Source: CAD feature listing. Evaluate the final solid. Frame: model axes, mm. A direction names the side the tool comes from. Give positions to 0.01 mm unless a question says otherwise; leave off trailing zeros. Order: outer loops, then holes, each group sorted by start corner. A loop starts at its lowest first (then second) coordinate and runs counter-clockwise, first axis right, second up. Notation, with made-up numbers: M 29.25,55 L 55.25,55 A22 ccw 55.25,93 Z; hole C 6,29.5 d10. An arc over 180 degrees is marked long. Use CSV: the item, a comma, the result in double quotes. Start each with the question number.
Item 1: Ray query, probe 1 along Y at (x, z) = (-76.2, 1.35) (3 decimals); probe 2 along Y at (x, z) = (-78, 2); probe 3 along Y at (x, z) = (-68, 1.45). Return the intervals inside material, ascending. Write a range as from..to.
Item 2: Section query C-C on y = 0. Return loops of the section in (x, z) (3 decimals), and give its area (3 significant figures).
Item 3: Access query for faces 1 (the face through (-7.651, 101.036, 1.252)), 2 (the face through (0.88, 71.75, 1.25)). Directions: +Z, -Z, +X, -X, +Y, -Y. A direction counts if a zero-diameter tool reaches every point of the face in a straight line with its end or side. Return the directions, or none.
Item 4: Section query B-B on x = -76.2. Return loops of the section in (y, z) (3 decimals).
Item 5: Section query A-A on z = 1.15. Return loops of the section in (x, y) (3 decimals), and give its area (3 significant figures).
Item 6: Pull-direction query (X, two-part tool) for faces 3 (the face through (-28, 42, 0)), 4 (the face through (-73.17, 0.95, 1.25)), 5 (the face through (0.304, 44.568, 1.252)); classes: +X half, -X half, draft (parallel to the pull), parting line (faces both ways), or undercut.
Item 7: First-contact query: pin 1 (1 mm diameter, centred on x = -26.5, z = 0.5, fed in from -Y); pin 2 (4 mm diameter, centred on x = -25.4, y = 101.6, fed in from +Z); pin 3 (1.5 mm diameter, centred on x = -63, z = 0.5, fed in from +Y); pin 4 (1.5 mm diameter, centred on x = -62, z = 2, fed in from +Y). Flat tips, straight axial feed; report the tip coordinate or a pass-through.
Item 8: Section query D-D on x = 0. Return loops of the section in (y, z) (3 decimals), and give its area (3 significant figures).
from build123d import *

# Parameters (mm, degrees)
SKETCH1_R           = 3.175
BOSS_EXTRUDE1_DEPTH = 2.54
FILLET1_R           = 3.81


with BuildPart() as part:
    # Sketch1 → Boss-Extrude1 (new body)
    with BuildSketch(Plane.XY):
        Polygon((-24.223713703, 118.151604251), (-88.735511623, -10.871991588), (8.032185257, 21.383907372), (-6.404519195, 64.694020727), (11.113552526, 81.656157748), align=None)
        with Locations((-76.2, 0)):
            Circle(SKETCH1_R, mode=Mode.SUBTRACT)
        with Locations((0, 25.4)):
            Circle(SKETCH1_R, mode=Mode.SUBTRACT)
        with Locations((-25.4, 101.6)):
            Circle(SKETCH1_R, mode=Mode.SUBTRACT)
    extrude(amount=BOSS_EXTRUDE1_DEPTH)

    # Fillet1
    fillet1_edges = [part.edges().sort_by_distance(p)[0] for p in [
        (11.113552526, 81.656157748, 1.27),
        (8.032185257, 21.383907372, 1.27),
        (-88.735511623, -10.871991588, 1.27),
    ]]
    fillet(fillet1_edges, radius=FILLET1_R)


solid = part.part
Verdict:
1,probe 1,"-6.693..-3.175, 3.175..14.199"
1,probe 2,"-7.29..-2.62, 2.62..10.6"
1,probe 3,"-3.96..30.6"
2,outline,"M -83.3,0 L -79.375,0 L -79.375,2.54 L -83.3,2.54 Z; M -73.025,0 L -56.12,0 L -56.12,2.54 L -73.025,2.54 Z"
2,area,"52.9 mm2"
3,face 1,"+Z, -Z, +X, +Y"
3,face 2,"+Z, -Z, +X"
4,outline,"M -6.693,0 L -3.175,0 L -3.175,2.54 L -6.693,2.54 Z; M 3.175,0 L 14.199,0 L 14.199,2.54 L 3.175,2.54 Z"
5,outline,"M -84.622,-2.645 A3.81 ccw -80.009,-7.963 L 4.418,20.179 A3.81 ccw 6.827,24.998 L -6.405,64.694 L 8.376,79.006 A3.81 ccw 8.463,84.393 L -24.224,118.152 Z; hole C -76.2,0 d6.35; hole C -25.4,101.6 d6.35; hole C 0,25.4 d6.35"
5,area,"5,700 mm2"
6,face 3,"draft"
6,face 4,"undercut"
6,face 5,"+X half"
7,pin 1,"y = 9.71"
7,pin 2,"through"
7,pin 3,"y = 42.1"
7,pin 4,"y = 44.1"
8,outline,"M 18.707,0 L 22.225,0 L 22.225,2.54 L 18.707,2.54 Z; M 28.575,0 L 45.48,0 L 45.48,2.54 L 28.575,2.54 Z; M 70.895,0 L 93.134,0 L 93.134,2.54 L 70.895,2.54 Z"
8,area,"108 mm2"
